Check sheet for the drawn part. Datum: minimum x, y, z corner. Units: mm. Give positions to 0.01 mm unless a question says otherwise; leave off trailing zeros. Write each loop counter-clockwise with the first axis right and the second up, starting at its lowest first coordinate (ties: lowest second). Pieces come first, ordered by that corner, then holes.
(1) Mould release check, pull along X, two halves, no side actions. Record for the marked faces 1 and 2: +X half, -X half, draft (parallel to the pull), parting line (faces both ways), or undercut.
(2) Cross-section at A-A (y = 35.5). Record the boundary of the cut face in (x, z), and give its area (3 significant figures).
(3) Thickness scan on line 1 along Z through (x, y) = (58.5, 56.5); line 2 along X through (y, z) = (278, 169.5); line 3 along X through (y, z) = (162.5, 61). Record the ranges inside material, lowest first.
(4) Depth check by flat-ended pin: P1, Ø1.5, axis at x = 65, y = 134.5, coming from the +Z side; P2, Ø10, axis at y = 196, z = 26, coming from the +X side; P3, Ø10, axis at x = 48.5, y = 123, coming from the -Z side. Enter the tip coordinate at first touch or a pass-through.
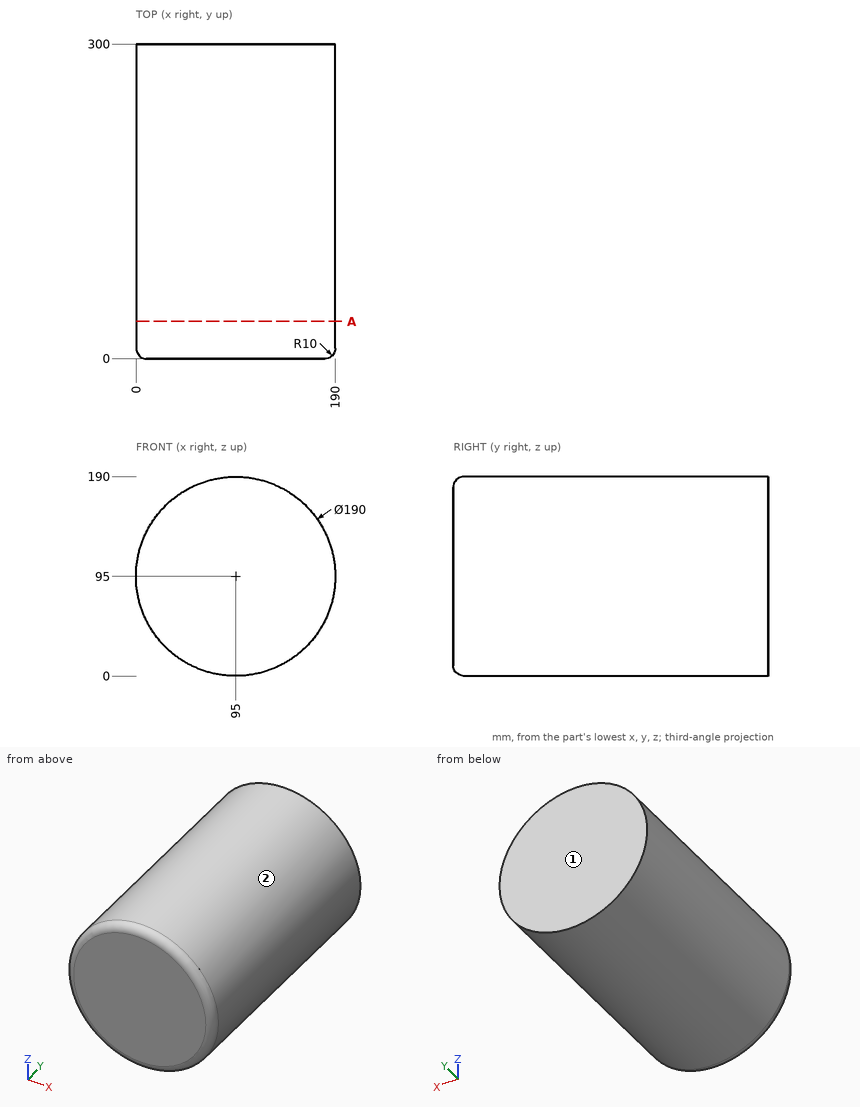
Reply:
1. face 1: draft
1. face 2: parting line
2. outline: circle Ø190 at (95, 95)
2. area: 28,400 mm2
3. line 1: z = 7.29 to 182.71
3. line 2: x = 36.05 to 153.95
3. line 3: x = 6.29 to 183.71
4. P1: stops at z = 185.38
4. P2: stops at x = 165.21
4. P3: stops at z = 9.54
